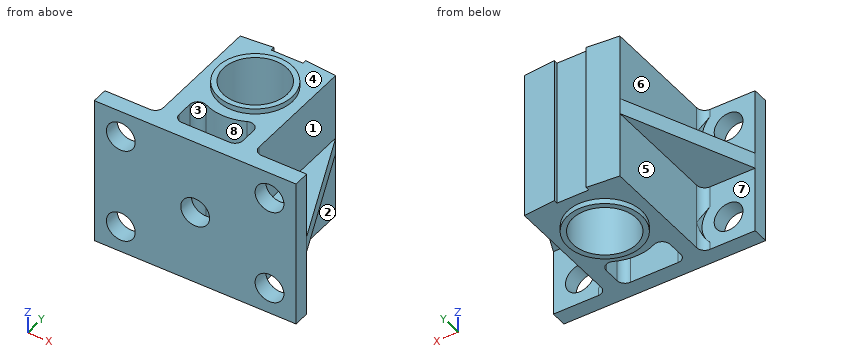
```python
from build123d import *

# Parameters (mm, degrees)
F0_R          = 4.7625
F1_DEPTH      = 22.225
F4_DEPTH      = 1.190625
F5_R          = 5.55625
F5_R_2        = 4.7625
F7_DEPTH      = 0.79375
F7_DEPTH_BACK = 23.01875
F8_R          = 1.7272
F9_DEPTH      = 10.0554862042
F11_DEPTH     = 22.225
F12_R         = 2.15265
F13_DEPTH     = 2.38125
F14_R         = 1.190625
F15_R         = 2.15265
F16_DEPTH     = 2.38125
F17_R         = 3.96875
F18_DEPTH     = 18.8729875805


with BuildPart() as f1:
    # F0 (on Top) → F1 (new body)
    with BuildSketch(Plane.XY):
        Polygon((-15.08125, -13.49375), (15.08125, -13.49375), (15.08125, -11.1125), (7.14375, -11.1125), (7.14375, 7.3428228204), (2.38125, 7.7594875805), (2.38125, 7.14375), (-2.38125, 7.14375), (-2.38125, 7.7594875805), (-7.14375, 7.3428228204), (-7.14375, -11.1125), (-15.08125, -11.1125), align=None)
        Circle(F0_R, mode=Mode.SUBTRACT)
    extrude(amount=F1_DEPTH)

    # F3 (on offset) → F4 (join, symmetric)
    with BuildSketch(Plane(origin=(0, 0, 11.1125), x_dir=(1, 0, 0), z_dir=(0, 0, -1))):
        Polygon((-15.08125, 11.1125), (-7.14375, -7.3428228204), (-7.14375, 11.1125), align=None)
        Polygon((15.08125, 11.1125), (7.14375, 11.1125), (7.14375, -7.3428228204), align=None)
    extrude(amount=F4_DEPTH, both=True)

    # F5 (on face) → F7 (join, two sides)
    with BuildSketch(Plane(origin=(0, 0, 0), x_dir=(1, 0, 0), z_dir=(0, 0, -1))) as f7_sk:
        Circle(F5_R)
        Circle(F5_R_2, mode=Mode.SUBTRACT)
    extrude(amount=F7_DEPTH)
    extrude(f7_sk.sketch, amount=-F7_DEPTH_BACK)

    # F8 (on face) → F9 (cut, up to face)
    with BuildSketch(Plane.XZ.offset(13.49375)):
        with Locations((0, 11.1125)):
            Circle(F8_R)
    extrude(amount=-F9_DEPTH, mode=Mode.SUBTRACT)

    # F10 (on face) → F11 (cut, through all)
    with BuildSketch(Plane.XY.offset(22.225)):
        with BuildLine():
            Line((-4.7625, -5.3246368714), (-4.7625, -11.1125))
            Line((-4.7625, -11.1125), (4.7625, -11.1125))
            Line((4.7625, -11.1125), (4.7625, -5.3246368714))
            ThreePointArc((4.7625, -5.3246368714), (0, -7.14375), (-4.7625, -5.3246368714))
        make_face()
    extrude(amount=-F11_DEPTH, mode=Mode.SUBTRACT)

    # F12 (on face) → F13 (cut, through all)
    with BuildSketch(Plane.XZ.offset(13.49375)):
        with Locations((0, 11.1125)):
            Circle(F12_R)
    extrude(amount=-F13_DEPTH, mode=Mode.SUBTRACT)

    # F14
    f14_edges = [f1.edges().sort_by_distance(p)[0] for p in [
        (7.14375, -11.1125, 4.960938),
        (7.14375, -11.1125, 17.264063),
        (-7.14375, -11.1125, 4.960938),
        (-7.14375, -11.1125, 17.264063),
        (-4.7625, -11.1125, 11.1125),
        (4.7625, -11.1125, 11.1125),
        (4.7625, -5.324637, 11.1125),
        (-4.7625, -5.324637, 11.1125),
    ]]
    fillet(f14_edges, radius=F14_R)

    # F15 (on face) → F16 (cut, through all)
    with BuildSketch(Plane.XZ.offset(13.49375)):
        with Locations((11.1125, 18.25625)):
            Circle(F15_R)
        with Locations((-11.1125, 18.25625)):
            Circle(F15_R)
        with Locations((-11.1125, 3.96875)):
            Circle(F15_R)
        with Locations((11.1125, 3.96875)):
            Circle(F15_R)
    extrude(amount=-F16_DEPTH, mode=Mode.SUBTRACT)

    # F17 (on face) → F18 (cut, through all)
    with BuildSketch(Plane(origin=(0, -11.1125, 0), x_dir=(-1, 0, 0), z_dir=(0, 1, 0))):
        with Locations((11.1125000001, 18.25625)):
            Circle(F17_R)
        with Locations((11.1125000001, 3.96875)):
            Circle(F17_R)
        with Locations((-11.1124999999, 3.96875)):
            Circle(F17_R)
        with Locations((-11.1124999999, 18.25625)):
            Circle(F17_R)
    extrude(amount=F18_DEPTH, mode=Mode.SUBTRACT)


solid = f1.part
```
Part model, mm, in its own coordinate system. Face numbers are marked on the shaded views. A direction names the side the tool comes from. Coordinates: 2 decimals unless noted, no trailing zeros. Write each loop counter-clockwise with the first axis right and the second up, starting at its lowest first coordinate (ties: lowest second). Pieces come first, ordered by that corner, then holes.
Item 1: Slice it at D-D (z = 8.25). Write the cut outline in (x, y) (1 decimal), and give its area (3 significant figures).
Item 2: Slice it at B-B (z = 17.5). Count the separate pieces of the cut face and the enclosed holes in it, and give its area (3 significant figures).
Item 3: Slice it at A-A (x = 0). Write the cut outline in (y, z) (1 decimal).
Item 4: Probe line 1 (Y direction, x = 0, z = 6.5); line 2 (X direction, y = 4.25, z = 20.75); line 3 (Z direction, x = 0, y = -11.85) (3 decimals). List the from-to ranges inside material, lowest first.
Item 5: Mould opens along X. For the marked faces 6, 7 and 8 say: released by +X, released by -X, zero draft, split by the parting line, or undercut.
Item 6: Pin check, flat tips, straight feed: pin 1 (2 mm diameter, centred on x = 0, z = 11.11, fed in from +Y); pin 2 (6 mm diameter, centred on x = -9, y = 1, fed in from -Z); pin 3 (2.5 mm diameter, centred on x = 12, y = -6, fed in from -Z); pin 4 (2.5 mm diameter, centred on x = 11.11, z = 3.97, fed in from -Y). Stop position of each tip, or through.
Item 7: Which spindle directions (+Z, -Z, +X, -X, +Y, -Y) get a long thin tool onto all of the face, cutting with end or side? Do the marked faces 1, 2, 3, 4 and 5. Say none if no direction does.
Item 8: Slice it at C-C (y = 0). Write the cut outline in (x, z) (1 decimal), and give its area (3 significant figures).
Results found:
1. outline: (-15.1, -13.5) - (15.1, -13.5) - (15.1, -11.1) - (8.3, -11.1) arc R1.2 cw to (7.1, -9.9) - (7.1, 7.3) - (2.4, 7.8) - (2.4, 7.1) - (-2.4, 7.1) - (-2.4, 7.8) - (-7.1, 7.3) - (-7.1, -9.9) arc R1.2 cw to (-8.3, -11.1) - (-15.1, -11.1) - close; hole (-4.8, -9.9) arc R1.2 ccw to (-3.6, -11.1) - (3.6, -11.1) arc R1.2 ccw to (4.8, -9.9) - (4.8, -7.5) arc R1.2 ccw to (3.1, -6.5) arc R7.1 cw to (-3.1, -6.5) arc R1.2 ccw to (-4.8, -7.5) - close; hole circle Ø9.5 at (0, 0)
1. area: 225 mm2
2. separate pieces: 3
2. enclosed holes: 2
2. area: 206 mm2
3. outline: (-13.5, 0) - (-11.1, 0) - (-11.1, 9) - (-13.5, 9) - close; (-13.5, 13.3) - (-11.1, 13.3) - (-11.1, 22.2) - (-13.5, 22.2) - close; (-7.1, 0) - (-5.6, 0) - (-5.6, -0.8) - (-4.8, -0.8) - (-4.8, 9.4) - (-7.1, 9.4) - close; (-7.1, 12.8) - (-4.8, 12.8) - (-4.8, 23) - (-5.6, 23) - (-5.6, 22.2) - (-7.1, 22.2) - close; (4.8, -0.8) - (5.6, -0.8) - (5.6, 0) - (7.1, 0) - (7.1, 22.2) - (5.6, 22.2) - (5.6, 23) - (4.8, 23) - close
4. line 1: y = -13.49 to -11.11, -7.14 to -4.76, 4.76 to 7.14
4. line 2: x = -7.14 to -2.15, 2.15 to 7.14
4. line 3: z = 0 to 8.96, 13.265 to 22.225
5. face 6: released by -X
5. face 7: zero draft
5. face 8: undercut
6. pin 1: stops at y = 7.14
6. pin 2: stops at z = 0
6. pin 3: stops at z = 9.92
6. pin 4: passes through
7. face 1: +Z, +X, +Y
7. face 2: -Z, +X, +Y
7. face 3: +Z, -Z
7. face 4: +Z
7. face 5: -Z, -X, +Y
8. outline: (-10.3, 9.9) - (-7.1, 9.9) - (-7.1, 0) - (-5.6, 0) - (-5.6, -0.8) - (-4.8, -0.8) - (-4.8, 23) - (-5.6, 23) - (-5.6, 22.2) - (-7.1, 22.2) - (-7.1, 12.3) - (-10.3, 12.3) - close; (4.8, -0.8) - (5.6, -0.8) - (5.6, 0) - (7.1, 0) - (7.1, 9.9) - (10.3, 9.9) - (10.3, 12.3) - (7.1, 12.3) - (7.1, 22.2) - (5.6, 22.2) - (5.6, 23) - (4.8, 23) - close
8. area: 123 mm2
